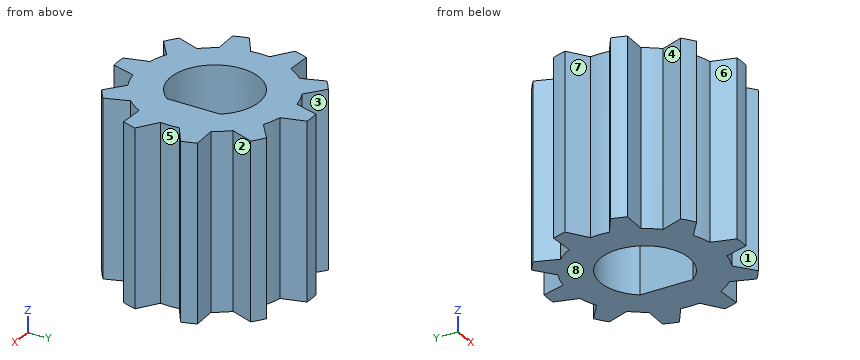
```python
from build123d import *

# Parameters (mm, degrees)
BOSS_EXTRUDE1_DEPTH = 10


with BuildPart() as part:
    # Sketch1 → Boss-Extrude1 (new body)
    with BuildSketch(Plane.XY):
        with BuildLine():
            Line((-0.796448866, 4.174705882), (-0.41969374, 5.483963636))
            ThreePointArc((-0.41969374, 5.483963636), (0, 5.5), (0.41969374, 5.483963636))
            Line((0.41969374, 5.483963636), (0.796448866, 4.174705882))
            ThreePointArc((0.796448866, 4.174705882), (1.313322226, 4.041990194), (1.809489883, 3.845548903))
            Line((1.809489883, 3.845548903), (2.883853582, 4.683309569))
            ThreePointArc((2.883853582, 4.683309569), (3.232818888, 4.449593469), (3.562932317, 4.189929988))
            Line((3.562932317, 4.189929988), (3.098171218, 2.909267108))
            ThreePointArc((3.098171218, 2.909267108), (3.438322226, 2.498087322), (3.724264998, 2.047522948))
            Line((3.724264998, 2.047522948), (5.085866854, 2.093790426))
            ThreePointArc((5.085866854, 2.093790426), (5.23081084, 1.699593469), (5.345251849, 1.295485494))
            Line((5.345251849, 1.295485494), (4.216497468, 0.53258718))
            ThreePointArc((4.216497468, 0.53258718), (4.25, 0), (4.216497468, -0.53258718))
            Line((4.216497468, -0.53258718), (5.345251849, -1.295485494))
            ThreePointArc((5.345251849, -1.295485494), (5.23081084, -1.699593469), (5.085866854, -2.093790426))
            Line((5.085866854, -2.093790426), (3.724264998, -2.047522948))
            ThreePointArc((3.724264998, -2.047522948), (3.438322226, -2.498087322), (3.098171218, -2.909267108))
            Line((3.098171218, -2.909267108), (3.562932317, -4.189929988))
            ThreePointArc((3.562932317, -4.189929988), (3.232818888, -4.449593469), (2.883853582, -4.683309569))
            Line((2.883853582, -4.683309569), (1.809489883, -3.845548903))
            ThreePointArc((1.809489883, -3.845548903), (1.313322226, -4.041990194), (0.796448866, -4.174705882))
            Line((0.796448866, -4.174705882), (0.41969374, -5.483963636))
            ThreePointArc((0.41969374, -5.483963636), (0, -5.5), (-0.41969374, -5.483963636))
            Line((-0.41969374, -5.483963636), (-0.796448866, -4.174705882))
            ThreePointArc((-0.796448866, -4.174705882), (-1.313322226, -4.041990194), (-1.809489883, -3.845548903))
            Line((-1.809489883, -3.845548903), (-2.883853582, -4.683309569))
            ThreePointArc((-2.883853582, -4.683309569), (-3.232818888, -4.449593469), (-3.562932317, -4.189929988))
            Line((-3.562932317, -4.189929988), (-3.098171218, -2.909267108))
            ThreePointArc((-3.098171218, -2.909267108), (-3.438322226, -2.498087322), (-3.724264998, -2.047522948))
            Line((-3.724264998, -2.047522948), (-5.085866854, -2.093790426))
            ThreePointArc((-5.085866854, -2.093790426), (-5.23081084, -1.699593469), (-5.345251849, -1.295485494))
            Line((-5.345251849, -1.295485494), (-4.216497468, -0.53258718))
            ThreePointArc((-4.216497468, -0.53258718), (-4.25, 0), (-4.216497468, 0.53258718))
            Line((-4.216497468, 0.53258718), (-5.345251849, 1.295485494))
            ThreePointArc((-5.345251849, 1.295485494), (-5.23081084, 1.699593469), (-5.085866854, 2.093790426))
            Line((-5.085866854, 2.093790426), (-3.724264998, 2.047522948))
            ThreePointArc((-3.724264998, 2.047522948), (-3.438322226, 2.498087322), (-3.098171218, 2.909267108))
            Line((-3.098171218, 2.909267108), (-3.562932317, 4.189929988))
            ThreePointArc((-3.562932317, 4.189929988), (-3.232818888, 4.449593469), (-2.883853582, 4.683309569))
            Line((-2.883853582, 4.683309569), (-1.809489883, 3.845548903))
            ThreePointArc((-1.809489883, 3.845548903), (-1.313322226, 4.041990194), (-0.796448866, 4.174705882))
        make_face()
        with BuildLine():
            Line((2, 1.5), (2, -1.5))
            ThreePointArc((2, -1.5), (-2.5, 0), (2, 1.5))
        make_face(mode=Mode.SUBTRACT)
    extrude(amount=BOSS_EXTRUDE1_DEPTH)


solid = part.part
```
Could you check a few things on this model? Use its own coordinates, in mm. Face numbers are marked on the shaded views. A direction names the side the tool comes from. Round coordinates to 2 decimals unless told otherwise and drop trailing zeros. Loops run counter-clockwise (first coordinate to the right, second up) from the corner with the lowest first, then second, coordinate; pieces in that order, holes last. Notation, with made-up numbers: M -4.5,-12.5 L 47.5,-12.5 A18 cw 47.5,14.5 Z; hole C 6,85 d7. An arc over 180 degrees is marked long. Write item = value, one per line.
1. I want a section at B-B, the plane x = 0. Write out the boundary of the cut face in (y, z).
Results below:
outline = M -5.5,0 L -2.5,0 L -2.5,10 L -5.5,10 Z; M 2.5,0 L 5.5,0 L 5.5,10 L 2.5,10 Z
2. I need wall thicknesses on probe 1 along Y at (x, z) = (0, 4.25); probe 2 along X at (y, z) = (0, 5.5); probe 3 along X at (y, z) = (4.25, 7.5). Which ranges of each line are inside material? Lowest first, please.
Results below:
probe_1 = -5.5 to -2.5, 2.5 to 5.5
probe_2 = -4.25 to -2.5, 2 to 4.25
probe_3 = -3.49 to -2.33, -0.77 to 0.77, 2.33 to 3.49
3. Thinking about a two-plate mould opening in X: for the marked faces 5, 6, 7 and 8, which applies, +X half, -X half, draft (parallel to the pull), parting line (faces both ways), or undercut?
Results below:
face_5 = +X half
face_6 = undercut
face_7 = -X half
face_8 = draft
4. Will these pins go through, and if not, where does the flat tip stop? P1, Ø3, axis at y = 2, z = 4, coming from the +X side; P2, Ø1.5, axis at x = 2, z = 5.5, coming from the +Y side; P3, Ø1.5, axis at x = 2, z = 5.5, coming from the -Y side.
Results below:
P1 = 5.35
P2 = 4.58
P3 = -4.58
5. I want a section at A-A, the plane y = 0. Write out the boundary of the cut face in (x, z).
Results below:
outline = M -4.25,0 L -2.5,0 L -2.5,10 L -4.25,10 Z; M 2,0 L 4.25,0 L 4.25,10 L 2,10 Z
6. Which directions (+Z, -Z, +X, -X, +Y, -Y) give clear straight access to the entire face, cutting with the end or side of a thin tool? Please do the marked faces 1, 2, 3 and 4.
Results below:
face_1 = +Z, -Z, -Y
face_2 = +Z, -Z, +X
face_3 = +Z, -Z, +Y
face_4 = +Z, -Z, -X
7. I want a section at C-C, the plane x = 3.25. Write out the boundary of the cut face in (y, z), and give its area (3 significant figures).
Results below:
outline = M -4.44,0 L -3.33,0 L -3.33,10 L -4.44,10 Z; M -2.74,0 L 2.74,0 L 2.74,10 L -2.74,10 Z; M 3.33,0 L 4.44,0 L 4.44,10 L 3.33,10 Z
area = 77.0 mm²
8. I want a section at D-D, the plane y = -4. Write out the boundary of the cut face in (x, z).
Results below:
outline = M -3.49,0 L -2.01,0 L -2.01,10 L -3.49,10 Z; M -1.44,0 L 1.44,0 L 1.44,10 L -1.44,10 Z; M 2.01,0 L 3.49,0 L 3.49,10 L 2.01,10 Z
